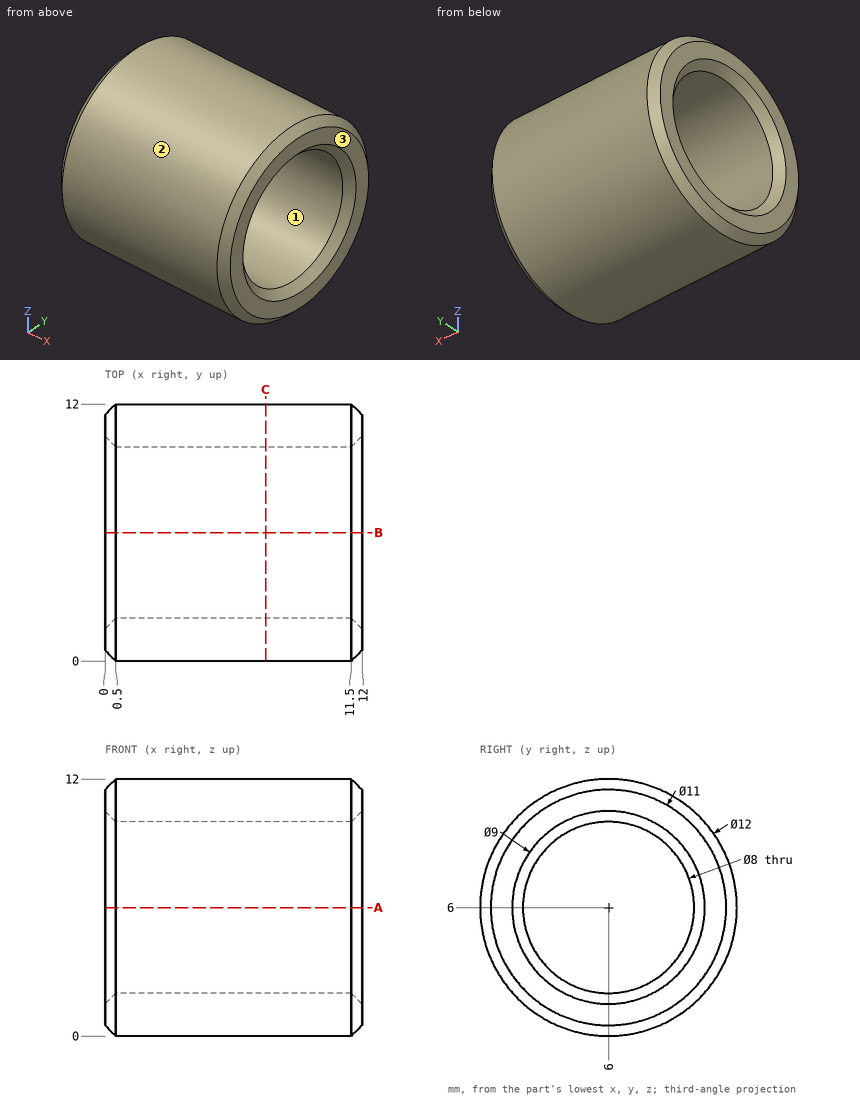
For this review, use the dimensioned drawing (mm, ordinates from the lowest corner) and the shaded views. Round coordinates to 2 decimals unless told otherwise and drop trailing zeros. Write each loop counter-clockwise with the first axis right and the second up, starting at its lowest first coordinate (ties: lowest second). Pieces come first, ordered by that corner, then holes. Notation, with made-up numbers: M 87,13.5 L 111,13.5 A23 ccw 111,43.5 Z; hole C -2.5,-27 d2. An arc over 180 degrees is marked long. Answer as CSV lines item,"result". Start each with the question number.
Q1. Consider section A-A, the plane z = 6. Give the boundary of the cut face in (x, y), then the cut area to 3 significant figures.
Q2. The part is to be moulded in two halves that separate along Y. For the marked faces 1, 2 and 3, say which applies: +Y half, -Y half, draft (parallel to the pull), parting line (faces both ways), or undercut.
Q3. Consider section C-C, the plane x = 7.5. Give the boundary of the cut face in (y, z).
Q4. Wall thickness on line 1 along Z through (x, y) = (8.75, 6); line 2 along Y through (x, z) = (6.5, 4.25); line 3 along Z through (x, y) = (5, 3): over which ranges is each line inside the solid? List them lowest first.
Q5. Clearance check with flat-ended pins moving along their axes: P1, Ø5, axis at y = 5, z = 7, coming from the -X side; P2, Ø1, axis at y = 2.5, z = 7.5, coming from the -X side; P3, Ø3, axis at x = 4, y = 8, coming from the -Z side; P4, Ø1.5, axis at x = 4.5, z = 2, coming from the -Y side. State where each tip first meets the part, or that it passes through.
Result set:
1,outline,"M 0,0.5 L 0.5,0 L 11.5,0 L 12,0.5 L 12,1.5 L 11.5,2 L 0.5,2 L 0,1.5 Z; M 0,10.5 L 0.5,10 L 11.5,10 L 12,10.5 L 12,11.5 L 11.5,12 L 0.5,12 L 0,11.5 Z"
1,area,"47.0 mm²"
2,face 1,"undercut"
2,face 2,"parting line"
2,face 3,"draft"
3,outline,"C 6,6 d12; hole C 6,6 d8"
4,line 1,"z = 0 to 2, 10 to 12"
4,line 2,"y = 0.26 to 2.4, 9.6 to 11.74"
4,line 3,"z = 0.8 to 3.35, 8.65 to 11.2"
5,P1,"passes through"
5,P2,"stops at x = 0.19"
5,P3,"stops at z = 0.02"
5,P4,"stops at y = 0.96"
